The listing builds one solid part. Answer for the finished solid, in the listing's coordinates (mm). A direction names the side the tool comes from. Round coordinates to 2 decimals unless told otherwise and drop trailing zeros. Loops run counter-clockwise (first coordinate to the right, second up) from the corner with the lowest first, then second, coordinate; pieces in that order, holes last. Notation, with made-up numbers: (20, 3) -> (37, 3) arc R15 ccw to (37, 32) -> close; hole circle Ø1 at (67.5, 38.25). An arc over 180 degrees is marked (long way). One line per question, with ' | ' between items.
from build123d import *

# Parameters (mm, degrees)
CHAMFER1_SIZE = 0.5
SKETCH3_W     = 1.5
SKETCH3_H     = 0.3


with BuildPart() as part:
    # Sketch1 → Revolve1 (revolve)
    with BuildSketch(Plane.XY, mode=Mode.PRIVATE) as revolve1_sk:
        Polygon((0, 0), (0, 7.5), (12, 7.5), (12, 9), (13, 10), (275, 10), (276, 9), (276, 7.5), (288, 7.5), (288, 5), (300, 5), (300, 0), align=None)
    revolve(revolve1_sk.sketch.rotate(Axis((0, 0, 0), (1, 0, 0)), 90), axis=Axis((0, 0, 0), (1, 0, 0)))

    # Chamfer1
    chamfer1_edges = [part.edges().sort_by_distance(p)[0] for p in [
        (288, 0, -7.5),
        (300, 0, -5),
        (0, 0, -7.5),
    ]]
    chamfer(chamfer1_edges, length=CHAMFER1_SIZE)

    # Sketch2 → Cut-Revolve1 (revolve, cut)
    with BuildSketch(Plane.XY, mode=Mode.PRIVATE) as cut_revolve1_sk:
        Polygon((0, 0), (0, 0.5), (0.5, 0), align=None)
        Polygon((300, 0), (300, 0.5), (299.5, 0), align=None)
    revolve(cut_revolve1_sk.sketch.rotate(Axis((0, 0, 0), (1, 0, 0)), 270), axis=Axis((0, 0, 0), (1, 0, 0)), mode=Mode.SUBTRACT)

    # Sketch3 → Cut-Revolve2 (revolve, cut)
    with BuildSketch(Plane.XY, mode=Mode.PRIVATE) as cut_revolve2_sk:
        with Locations((11.25, 7.35)):
            Rectangle(SKETCH3_W, SKETCH3_H)
        with Locations((276.75, 7.35)):
            Rectangle(SKETCH3_W, SKETCH3_H)
        with Locations((288.75, 4.85)):
            Rectangle(SKETCH3_W, SKETCH3_H)
    revolve(cut_revolve2_sk.sketch.rotate(Axis((0, 0, 0), (1, 0, 0)), 90), axis=Axis((0, 0, 0), (1, 0, 0)), mode=Mode.SUBTRACT)


solid = part.part
Q1. Find the intervals of material crossed by line 1 (X direction, y = -1.5, z = 7.75); line 2 (Y direction, x = 151, z = 0.5); line 3 (Y direction, x = 112, z = -4.25), in increasing order. Write a range as from..to.
Numbers:
line 1: 12..276 | line 2: -9.99..9.99 | line 3: -9.05..9.05
Q2. A cutting plane is placed at A-A on x = 171. Give the vertices of the cut face in (y, z), plus the area to 3 significant figures.
Numbers:
outline: circle Ø20 at (0, 0) | area: 314 mm^2
Q3. For faces 1 (the face through (282.57, -6.324, 4.032)), 2 (the face through (5.57, -6.324, 4.032)), 3 (the face through (288.76, 4.17, 2.17)), determine the directions among +Z, -Z, +X, -X, +Y, -Y from which every point of the face is accessible in a straight line to the end or side of a thin tool.
Numbers:
face 1: +X | face 2: -X | face 3: none
Q4. Given pin 1 Ø5 at (x, y) = (206.5, 5.5) entering from -Z; pin 2 Ø12 at (y, z) = (-1, 2) entering from -X; pin 3 Ø1 at (y, z) = (3.5, 5.5) entering from +X; pin 4 Ø4 at (x, y) = (180, -6.5) entering from +Z, each flat-ended and moving along its own axis, determine where each tip first touches the part or whether it passes through.
Numbers:
pin 1: z = -9.54 | pin 2: x = 0 | pin 3: x = 288 | pin 4: z = 8.93
